For this review, use the dimensioned drawing (mm, ordinates from the lowest corner) and the shaded views. A direction names the side the tool comes from. Coordinates: 2 decimals unless noted, no trailing zeros. Loops run counter-clockwise (first coordinate to the right, second up) from the corner with the lowest first, then second, coordinate; pieces in that order, holes last. Notation, with made-up numbers: M 73,-23.75 L 110,-23.75 A29 ccw 110,-1.75 Z; hole C 43.25,52.25 d1. An arc over 180 degrees is marked long. Write item = value, one per line.
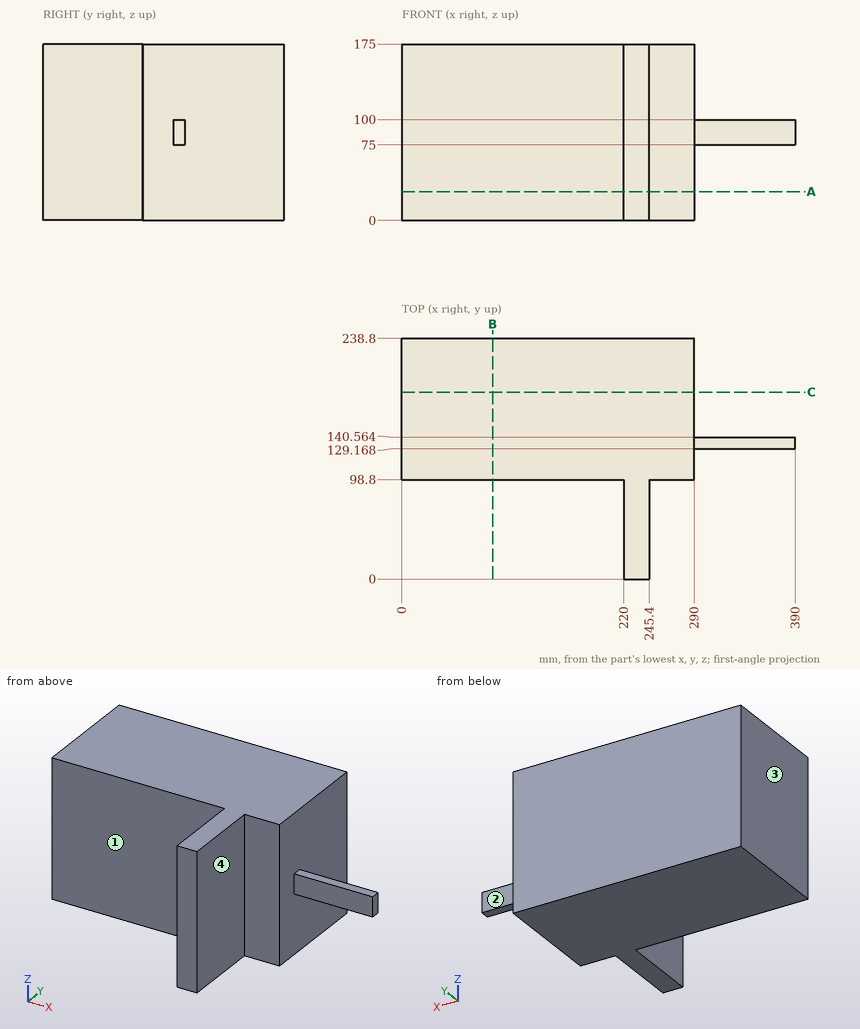
Q1. For pin 1 Ø7.5 at (x, z) = (356, 86) entering from +Y; pin 2 Ø3.5 at (x, y) = (333, 135) entering from -Z; pin 3 Ø12.5 at (x, z) = (333, 88.5) entering from -Y, all flat-tipped, find the tip position at first contact; note any pin that passes through.
Solved:
pin_1 = 140.56
pin_2 = 75
pin_3 = 129.17
Q2. Add section B-B (x = 90). Write out the cut boundary in (y, z).
Solved:
outline = M 98.8,0 L 238.8,0 L 238.8,175 L 98.8,175 Z
Q3. For line 1 along X through (y, z) = (127.5, 13); line 2 along X through (y, z) = (89, 160.5); line 3 along Y through (x, z) = (207, 91), list the stretches that pass through material, from the lowest coordinate up.
Solved:
line_1 = 0 to 290
line_2 = 220 to 245.4
line_3 = 98.8 to 238.8
Q4. Add section C-C (y = 185.5). Write out the cut boundary in (x, z), and give its area (4 significant figures).
Solved:
outline = M 0,0 L 290,0 L 290,175 L 0,175 Z
area = 50,750 mm²
Q5. Machinability: for the marked faces 1, 2, 3 and 4, which of the approach directions +Z, -Z, +X, -X, +Y, -Y give a long, thin tool a straight path to every point of the face, cutting with its end or side? Answer none if there is none.
Solved:
face_1 = +Z, -Z, -X, -Y
face_2 = +Z, -Z, +X, +Y
face_3 = +Z, -Z, -X, +Y, -Y
face_4 = +Z, -Z, +X, -Y
Q6. Add section A-A (z = 28.5). Write out the cut boundary in (x, y).
Solved:
outline = M 0,98.8 L 220,98.8 L 220,0 L 245.4,0 L 245.4,98.8 L 290,98.8 L 290,238.8 L 0,238.8 Z
